Geometry check sheet. Reference: the model listing, model coordinates, mm. A direction names the side the tool comes from. Round coordinates to 2 decimals unless told otherwise and drop trailing zeros. Order: outer loops, then holes, each group sorted by start corner. A loop starts at its lowest first (then second) coordinate and runs counter-clockwise, first axis right, second up. Notation, with made-up numbers: (68, -24) - (106, -24) arc R29 cw to (106, -3) - close; hole circle Ø1 at (-11, -21). An arc over 180 degrees is marked (long way). Return JSON: item names as keys, results as strings. Group by question number.
Q1. Sectioned sample at C-C, the plane z = -228. Record the cut outline in (x, y).
Q2. Sectioned sample at A-A, the plane z = -251.5. Record the cut outline in (x, y), then the cut area to 3 significant figures.
Q3. Sectioned sample at D-D, the plane x = 155. Record the cut outline in (y, z), then the cut area to 3 significant figures.
Q4. Gauge pin test, flat end, axial feed: pin 1 Ø5 at (x, z) = (78.66, -216.13) entering from -Y. Record the tip position at first contact, or that the pin passes through.
Q5. Tool access check on faces 1 (the cylindrical face through (60.416, 2.465, -148.155)), 2 (the flat face through (127, 2, -127)), 3 (the flat face through (131.64, 2.465, -143.514)), 4 (the flat face through (168.51, 2.46, -184.45)), 5 (the flat face through (105.436, 2.465, -181.629)). Record the directions out of +Z, -Z, +X, -X, +Y, -Y that give a thin tool (end or side, any length) a straight path to the whole face; none if there is none.
Q6. Material ranges on line 1 along X through (y, z) = (2.05, -191.5); line 2 along X through (y, z) = (2.4, -202); line 3 along Z through (x, y) = (107, 4.4), recorded low to high.
Q7. Sectioned sample at B-B, the plane y = 4.1. Give the number of separate pieces and of enclosed holes in the cut face, then the cut area to 3 significant figures.
Autodesk Inventor part; units mm, degrees
ref_plane "YZ Plane" through (0, 0, 0) normal (1, 0, 0) x (0, 1, 0)
ref_plane "XZ Plane" through (0, 0, 0) normal (0, 1, 0) x (-1, 0, 0)
ref_plane "XY Plane" through (0, 0, 0) normal (0, 0, 1) x (1, 0, 0)
sketch "Sketch2" plane through (0, 0, 0) normal (0, 1, 0) x (-1, 0, 0)
  circle A0 centre (0, 0) radius 285
  circle A1 centre (0, 0) radius 160
  line L0 (0, 0) -> (0, -285)
  line L1 (0, 0) -> (-201.5254, -201.5254)
  line L2 (0, 0) -> (24.8394, -283.9155)
  line L3 (0, 0) -> (-183.1945, -218.3227)
  circle A2 centre (0, 0) radius 255
  circle A3 centre (0, 0) radius 190
  circle A4 centre (0, 0) radius 200
  circle A5 centre (0, 0) radius 245
  line L4 (16.5596, -189.277) -> (0, -200)
  line L5 (22.2247, -254.0296) -> (0, -245)
  line L6 (-122.1296, -145.5484) -> (-141.4214, -141.4214)
  line L7 (-163.9108, -195.3413) -> (-173.2412, -173.2412)
  line L8 (-123.7453, -217.2835) -> (-128.0398, -214.7227)
  line L9 (-128.0398, -214.7227) -> (-107.5534, -180.367)
  line L10 (-107.5534, -180.367) -> (-103.2589, -182.9278)
  line L11 (-103.2589, -182.9278) -> (-123.7453, -217.2835)
  line L12 (-123.7453, -217.2835) -> (-107.5534, -180.367) construction
  line L13 (-128.0398, -214.7227) -> (-103.2589, -182.9278) construction
  circle A6 centre (0, 0) radius 230 construction
  line L14 (0, 0) -> (-97.4757, -267.8124) construction
  circle A7 centre (0, 0) radius 210 construction
  circle A8 centre (0, 0) radius 250 construction
  line L15 (-44.8727, -245.9907) -> (-39.9369, -246.7895)
  line L16 (-39.9369, -246.7895) -> (-33.547, -207.3032)
  line L17 (-33.547, -207.3032) -> (-38.4828, -206.5044)
  line L18 (-38.4828, -206.5044) -> (-44.8727, -245.9907)
  line L19 (-44.8727, -245.9907) -> (-33.547, -207.3032) construction
  line L20 (-39.9369, -246.7895) -> (-38.4828, -206.5044) construction
  circle A9 centre (-78.6646, -216.1293) radius 4
  point P0 (-115.6493, -198.8252)
  point P1 (0, -160)
  point P2 (-113.1371, -113.1371)
  dimension "d0" = 570
  dimension "d1" = 320
  dimension "d2" = 45
  dimension "d3" = 5
  dimension "d4" = 5
  dimension "d5" = 30
  dimension "d6" = 30
  dimension "d7" = 10
  dimension "d8" = 10
  dimension "d11" = 5
  dimension "d14" = 20
  dimension "d19" = 39.2099
  dimension "d20" = 40
  dimension "d21" = 50
  dimension "d24" = 8
  dimension "d35" = 70
extrude "Extrusion1" add sketch "Sketch2" along normal blind 5 contours L1 A2 L3 A0 | L3 A2 L0 A0 | L1 L7 A2 | L5 A5 L2 | L3 A5 L9 L8 L11 L18 L15 L16 L0 A2 | A5 L0 A4 L2 | A5 L16 L17 L18 L11 L10 L9 L3 A4 L0 | L1 A3 L6 | A4 L4 L2 | A4 L3 A3 L0 | L1 A1 L3 A3 | L3 A1 L0 A3
sketch "Sketch3" plane through (0, 5, 0) normal (0, 1, 0) x (1, 0, 0)
  circle A0 centre (0, 0) radius 185
  circle A1 centre (0, 0) radius 265
  point P0 (94.9402, 247.4093)
  point P1 (66.3297, 172.7002)
  point P2 (16.7015, 184.2446)
  point P3 (24.8728, 263.8301)
  point P4 (110.6548, 148.2583)
  point P5 (158.2673, 212.5475)
  dimension "d32" = 370
  dimension "d34" = 530
hole "Hole1" at (94.9402, 5, -247.4093) at (66.3297, 5, -172.7002) at (16.7015, 5, -184.2446) at (24.8728, 5, -263.8301) at (110.6548, 5, -148.2583) at (158.2673, 5, -212.5475) direction (0, -1, 0) diameter 1.778 end through all
properties part number "Non-Rotating Carousel Plate" material "PLA 33 Plastic"
Reply:
{
 "1": {"outline": "(-19.95, 0) - (36.9, 0) - (36.9, 5) - (-19.95, 5) - close; (41.96, 0) - (171, 0) - (171, 5) - (41.96, 5) - close"},
 "2": {"outline": "(-22, 0) - (-16, 0) - (-16, 5) - (-22, 5) - close; (0, 0) - (134.06, 0) - (134.06, 5) - (0, 5) - close", "area": "700 mm^2"},
 "3": {"outline": "(0, -239.17) - (5, -239.17) - (5, -184.72) - (0, -184.72) - close", "area": "272 mm^2"},
 "4": {"pin 1": "through"},
 "5": {"face 1": "+Z, -X, +Y, -Y", "face 2": "+Z, +X, +Y, -Y", "face 3": "+X, +Y, -Y", "face 4": "+Z, +Y, -Y", "face 5": "+Y, -Y"},
 "6": {"line 1": "-16.75 to -13.13, 0 to 108.37, 114.19 to 160.69, 165.53 to 191.5", "line 2": "-17.67 to 114.63, 120.45 to 201.05", "line 3": "-264.15 to -189.2, -180.7 to -118.96"},
 "7": {"separate pieces": "1", "enclosed holes": "9", "area": "21,400 mm^2"}
}
